Model file for the job. Use its own axes, mm. A direction names the side the tool comes from. Give positions to 0.01 mm unless a question says otherwise; leave off trailing zeros. Loops run counter-clockwise (first coordinate to the right, second up) from the corner with the lowest first, then second, coordinate; pieces in that order, holes last. Notation, with made-up numbers: (18.25, -37.5) - (46.25, -37.5) arc R23 ccw to (46.25, 1.5) - close; hole circle Ø6 at (16.25, 83). An arc over 180 degrees is marked (long way). Use a Markdown table: item, result.
from build123d import *

# Parameters (mm, degrees)
SKETCH1_W           = 508
SKETCH1_H           = 635
BOSS_EXTRUDE1_DEPTH = 6.35
SKETCH2_R           = 6.35
BOSS_EXTRUDE2_DEPTH = 177.8
SKETCH3_W           = 508
SKETCH3_H           = 298.45
BOSS_EXTRUDE3_DEPTH = 6.35
BOSS_EXTRUDE4_DEPTH = 12.7
SKETCH6_W           = 298.45
SKETCH6_H           = 25.4
BOSS_EXTRUDE6_DEPTH = 482.6
CUT_EXTRUDE1_DEPTH  = 25.4


with BuildPart() as part:
    # Sketch1 → Boss-Extrude1 (new body)
    with BuildSketch(Plane.XY):
        with Locations((254, 317.5)):
            Rectangle(SKETCH1_W, SKETCH1_H)
    extrude(amount=BOSS_EXTRUDE1_DEPTH)

    # Sketch2 → Boss-Extrude2 (add)
    with BuildSketch(Plane.XY):
        with Locations(Location((254, 203.2, 0), (0, 0, 180))):
            Circle(SKETCH2_R)
    extrude(amount=BOSS_EXTRUDE2_DEPTH)

    # Sketch3 → Boss-Extrude3 (add)
    with BuildSketch(Plane(origin=(0, 0, 0), x_dir=(1, 0, 0), z_dir=(0, 1, 0))):
        with Locations((254, -155.575)):
            Rectangle(SKETCH3_W, SKETCH3_H)
    extrude(amount=BOSS_EXTRUDE3_DEPTH)

    # Sketch4 → Boss-Extrude4 (add)
    with BuildSketch(Plane(origin=(0, 0, 0), x_dir=(0, 0, -1), z_dir=(1, 0, 0))):
        Polygon((-304.8, 6.35), (-304.8, 635), (-6.35, 635), (-6.35, 609.6), (-279.4, 609.6), (-279.4, 6.35), align=None)
    boss_extrude4 = extrude(amount=BOSS_EXTRUDE4_DEPTH)

    # Mirror1: Boss-Extrude4 across plane
    add(boss_extrude4.mirror(Plane(origin=(254, 0, 0), x_dir=(0, 0, 1), z_dir=(1, 0, 0))))

    # Sketch6 → Boss-Extrude6 (add)
    with BuildSketch(Plane(origin=(12.7, 0, 0), x_dir=(0, 0, -1), z_dir=(1, 0, 0))):
        with Locations((-155.575, 622.3)):
            Rectangle(SKETCH6_W, SKETCH6_H)
    extrude(amount=BOSS_EXTRUDE6_DEPTH)

    # Sketch7 → Cut-Extrude1 (cut)
    with BuildSketch(Plane(origin=(0, 635, 0), x_dir=(1, 0, 0), z_dir=(0, 1, 0))):
        with BuildLine():
            Line((292.1, -63.5), (292.1, -241.3))
            ThreePointArc((292.1, -241.3), (254, -279.4), (215.9, -241.3))
            Line((215.9, -241.3), (215.9, -63.5))
            ThreePointArc((215.9, -63.5), (254, -25.4), (292.1, -63.5))
        make_face()
    extrude(amount=-CUT_EXTRUDE1_DEPTH, mode=Mode.SUBTRACT)


solid = part.part
(1) Slice it at C-C, the plane x = 409. Write the cut outline in (y, z), plus the area to 3 significant figures.
Computed:
| item | result |
|---|---|
| outline | (0, 0) - (635, 0) - (635, 304.8) - (609.6, 304.8) - (609.6, 6.35) - (6.35, 6.35) - (6.35, 304.8) - (0, 304.8) - close |
| area | 13,500 mm² |
(2) Slice it at A-A, the plane y = 439. Write the cut outline in (x, z), plus the area to 3 significant figures.
Computed:
| item | result |
|---|---|
| outline | (0, 0) - (508, 0) - (508, 6.35) - (0, 6.35) - close; (0, 279.4) - (12.7, 279.4) - (12.7, 304.8) - (0, 304.8) - close; (495.3, 279.4) - (508, 279.4) - (508, 304.8) - (495.3, 304.8) - close |
| area | 3,870 mm² |
(3) Drill centre lines: probe 1 along Y at (x, z) = (400.5, 243); probe 2 along X at (y, z) = (415, 288); probe 3 along Z at (x, y) = (26, 329). Where is each one in solid material? Low to high. Write a range as [from, to].
Computed:
| item | result |
|---|---|
| probe 1 | [0, 6.35], [609.6, 635] |
| probe 2 | [0, 12.7], [495.3, 508] |
| probe 3 | [0, 6.35] |
(4) Slice it at B-B, the plane z = 79.5. Write the cut outline in (x, y), plus the area to 3 significant figures.
Computed:
| item | result |
|---|---|
| outline | (0, 0) - (508, 0) - (508, 6.35) - (0, 6.35) - close; (0, 609.6) - (215.9, 609.6) - (215.9, 635) - (0, 635) - close; circle Ø12.7 at (254, 203.2); (292.1, 609.6) - (508, 609.6) - (508, 635) - (292.1, 635) - close |
| area | 14,300 mm² |
(5) Pin check, flat tips, straight feed: P1, Ø10, axis at x = 277.5, z = 104, coming from the +Y side; P2, Ø10, axis at x = 76, y = 108.5, coming from the +Z side; P3, Ø4, axis at x = 254, y = 206.5, coming from the +Z side. Stop position of each tip, or through.
Computed:
| item | result |
|---|---|
| P1 | y = 6.35 |
| P2 | z = 6.35 |
| P3 | z = 177.8 |
(6) Slice it at D-D, the plane x = 226.5. Write the cut outline in (y, z).
Computed:
| item | result |
|---|---|
| outline | (0, 0) - (635, 0) - (635, 37.13) - (609.6, 37.13) - (609.6, 6.35) - (6.35, 6.35) - (6.35, 304.8) - (0, 304.8) - close; (609.6, 267.67) - (635, 267.67) - (635, 304.8) - (609.6, 304.8) - close |
(7) Mould opens along X. For faces 1 (the flat face through (250, 0, 150)), 2 (the flat face through (292.1, 622, 151)), 3 (the flat face through (508, 390, 287)) say: pulls with the +X half, pulls with the -X half, needs draft (parallel to the pull), parting line crosses it, or undercut.
Computed:
| item | result |
|---|---|
| face 1 | needs draft |
| face 2 | undercut |
| face 3 | pulls with the +X half |
(8) 3-axis set-ups, long thin cutter, end or side, ignore diameter. For faces 4 (the flat face through (194, 635, 155)), 5 (the flat face through (495.3, 312, 292)), 6 (the flat face through (215.9, 622, 154)): which of +Z, -Z, +X, -X, +Y, -Y reach the whole face in a straight line?
Computed:
| item | result |
|---|---|
| face 4 | +Z, -Z, +X, -X, +Y |
| face 5 | +Z |
| face 6 | +Y |
